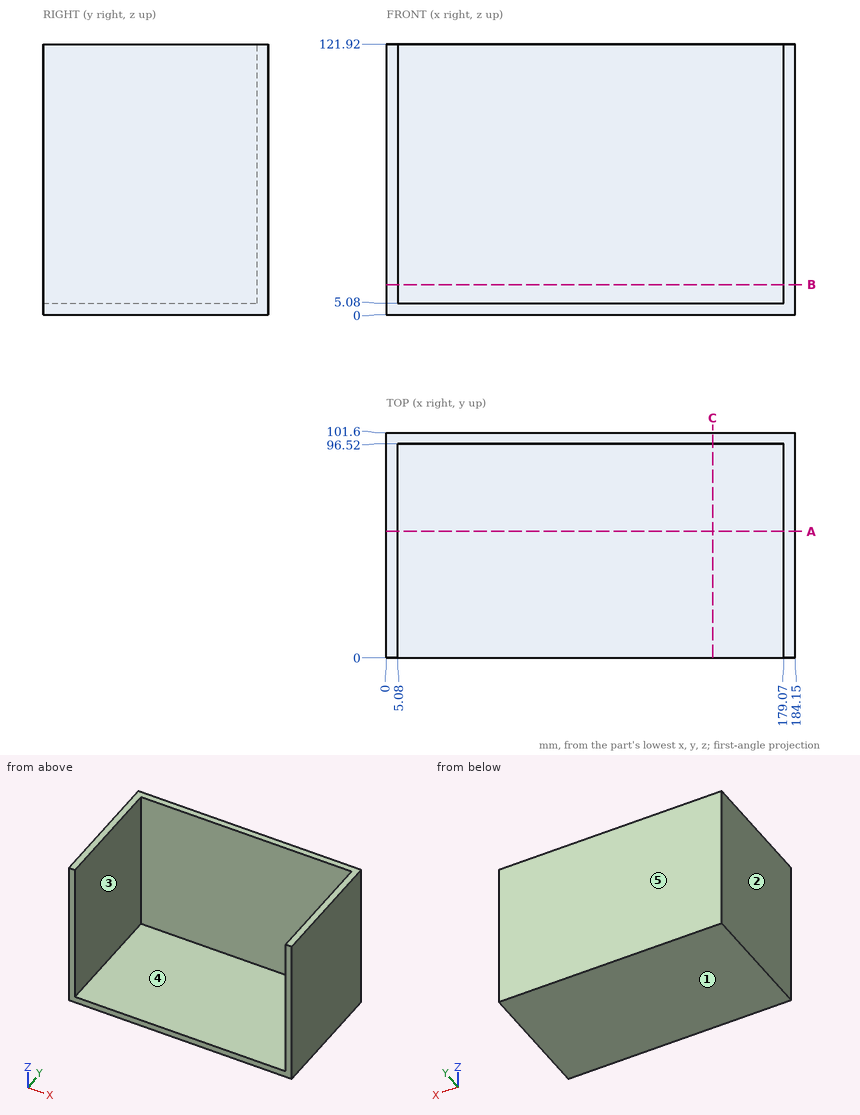
Input: dimensioned drawing with shaded views. Units: mm. Origin: part minimum x, y, z. A direction names the side the tool comes from. Coordinates: 2 decimals unless noted, no trailing zeros. Write each loop counter-clockwise with the first axis right and the second up, starting at its lowest first coordinate (ties: lowest second). Pieces come first, ordered by that corner, then holes. Notation, with made-up numbers: M 61.5,8 L 104.5,8 A21 ccw 104.5,41 Z; hole C 67.25,46 d4. An arc over 180 degrees is marked long. Answer as CSV lines item,"result". Start each with the question number.
Q1. Reachability of the marked faces 4 and 5 from +Z, -Z, +X, -X, +Y, -Y: full face, straight path, thin tool, end or side. Return the list, or none.
Q2. Cut plane A-A on y = 57. Return the cut outline in (x, z), then the cut area to 3 significant figures.
Q3. Pin query (flat end, axial travel): P1, Ø8, axis at x = 165, y = 74, coming from the +Z side; P2, Ø2, axis at x = 21, z = 97, coming from the -Y side. Return the tip coordinate at first contact, or that it passes through.
Q4. Mould query, pull axis X, two halves, no side actions, for the marked faces 1, 2 and 3. Classes: released by +X, released by -X, zero draft, split by the parting line, or undercut.
Q5. Line query: line 1 (X direction, y = 36.5, z = 113.5); line 2 (Z direction, x = 62.5, y = 71); line 3 (Y direction, x = 127, z = 45). Output: solid intervals per line, ascending. Write a range as from..to.
Q6. Cut plane B-B on z = 13.5. Return the cut outline in (x, y), then the cut area to 3 significant figures.
Q7. Cut plane C-C on x = 147. Return the cut outline in (y, z), then the cut area to 3 significant figures.
Findings below:
1,face 4,"+Z, -Y"
1,face 5,"+Z, -Z, +X, -X, +Y"
2,outline,"M 0,0 L 184.15,0 L 184.15,121.92 L 179.07,121.92 L 179.07,5.08 L 5.08,5.08 L 5.08,121.92 L 0,121.92 Z"
2,area,"2,120 mm2"
3,P1,"stops at z = 5.08"
3,P2,"stops at y = 96.52"
4,face 1,"zero draft"
4,face 2,"released by -X"
4,face 3,"undercut"
5,line 1,"x = 0..5.08, 179.07..184.15"
5,line 2,"z = 0..5.08"
5,line 3,"y = 96.52..101.6"
6,outline,"M 0,0 L 5.08,0 L 5.08,96.52 L 179.07,96.52 L 179.07,0 L 184.15,0 L 184.15,101.6 L 0,101.6 Z"
6,area,"1,920 mm2"
7,outline,"M 0,0 L 101.6,0 L 101.6,121.92 L 96.52,121.92 L 96.52,5.08 L 0,5.08 Z"
7,area,"1,110 mm2"
